```python
from build123d import *

# Parameters (mm, degrees)
SKETCH133_W     = 50
SKETCH133_H     = 100
SKETCH133_R     = 1.9
SKETCH133_R_2   = 1.75
PAD079_DEPTH    = 10
SKETCH143_R     = 2.5
POCKET049_DEPTH = 2
SKETCH149_R     = 1.73
POCKET051_DEPTH = 10


with BuildPart() as part:
    # Sketch133 → Pad079 (new body)
    with BuildSketch(Plane.XY):
        Rectangle(SKETCH133_W, SKETCH133_H)
        with Locations((-10, 40)):
            Circle(SKETCH133_R, mode=Mode.SUBTRACT)
        with Locations((10, 40)):
            Circle(SKETCH133_R, mode=Mode.SUBTRACT)
        with Locations((10, 20)):
            Circle(SKETCH133_R, mode=Mode.SUBTRACT)
        with Locations((-10, 20)):
            Circle(SKETCH133_R, mode=Mode.SUBTRACT)
        with Locations((-10, -20)):
            Circle(SKETCH133_R, mode=Mode.SUBTRACT)
        with Locations((10, -20)):
            Circle(SKETCH133_R, mode=Mode.SUBTRACT)
        with Locations((10, -40)):
            Circle(SKETCH133_R, mode=Mode.SUBTRACT)
        with Locations((-10, -40)):
            Circle(SKETCH133_R, mode=Mode.SUBTRACT)
        with Locations((12.5, 0)):
            Circle(SKETCH133_R_2, mode=Mode.SUBTRACT)
        with Locations((-12.5, 0)):
            Circle(SKETCH133_R_2, mode=Mode.SUBTRACT)
        with Locations((20, 40)):
            Circle(SKETCH133_R_2, mode=Mode.SUBTRACT)
        with Locations((20, 20)):
            Circle(SKETCH133_R_2, mode=Mode.SUBTRACT)
        with Locations((-20, 40)):
            Circle(SKETCH133_R_2, mode=Mode.SUBTRACT)
        with Locations((-20, 20)):
            Circle(SKETCH133_R_2, mode=Mode.SUBTRACT)
        with Locations((-20, -20)):
            Circle(SKETCH133_R_2, mode=Mode.SUBTRACT)
        with Locations((-20, -40)):
            Circle(SKETCH133_R_2, mode=Mode.SUBTRACT)
        with Locations((20, -20)):
            Circle(SKETCH133_R_2, mode=Mode.SUBTRACT)
        with Locations((20, -40)):
            Circle(SKETCH133_R_2, mode=Mode.SUBTRACT)
    extrude(amount=PAD079_DEPTH)

    # Sketch143 → Pocket049 (cut)
    with BuildSketch(Plane.YZ.offset(25)):
        with Locations((-45, 5)):
            Circle(SKETCH143_R)
        with Locations((45, 5)):
            Circle(SKETCH143_R)
    extrude(amount=-POCKET049_DEPTH, mode=Mode.SUBTRACT)

    # Sketch149 → Pocket051 (cut)
    with BuildSketch(Plane.YZ.offset(-25)):
        with Locations((-10, 5)):
            Circle(SKETCH149_R)
        with Locations((10, 5)):
            Circle(SKETCH149_R)
    extrude(amount=POCKET051_DEPTH, mode=Mode.SUBTRACT)


solid = part.part
```
The model under review builds one solid part; all positions refer to its coordinate system, in mm. A direction names the side the tool comes from. Coordinates: 2 decimals unless noted, no trailing zeros. Write each loop counter-clockwise with the first axis right and the second up, starting at its lowest first coordinate (ties: lowest second). Pieces come first, ordered by that corner, then holes. Notation, with made-up numbers: (57.25, 37.5) -> (73.25, 37.5) arc R24 cw to (73.25, 47.5) -> close; hole circle Ø9 at (-7, 10.5). An arc over 180 degrees is marked (long way). One line per item, written item: value. Start each with the question number.
Q1. Add section C-C, the plane x = 20. Give the boundary of the cut face in (y, z).
Q2. Add section B-B, the plane y = 20. Give the boundary of the cut face in (x, z), then the cut area to 3 significant figures.
Q3. Add section A-A, the plane x = -20. Give the boundary of the cut face in (y, z), then the cut area to 3 significant figures.
Q4. For faces 1 (the face through (23, 45, 5)), 2 (the face through (-15, -10, 5)), 3 (the face through (0, 50, 5)), list the 3-axis set-ups (+Z, -Z, +X, -X, +Y, -Y) from which the entire face can be reached by the end or side of a thin tool; tool diameter is ignored.
Q5. To check wall thickness, follow probe 1 along Y at (x, z) = (10, 6); probe 2 along Y at (x, z) = (20, 3.25); probe 3 along Y at (x, z) = (12.5, 5.25). State the ranges of each line that lie inside material, in increasing order.
Q6. Add section D-D, the plane y = 10. Give the boundary of the cut face in (x, z), then the cut area to 3 significant figures.
Q7. Clearance check with flat-ended pins moving along their axes: P1, Ø3, axis at y = -10, z = 5, coming from the -X side; P2, Ø1.5, axis at y = -44.5, z = 4, coming from the +X side. State where each tip first meets the part, or that it passes through.
Q8. The part is to be moulded in two halves that separate along Z. For faces 4 (the face through (24.01, 47.31, 4.04)), 5 (the face through (0, 1, 10)), 6 (the face through (18.61, 38.94, 4.93)), 7 (the face through (0, 1, 0)), say which applies: +Z half, -Z half, draft (parallel to the pull), parting line (faces both ways), or undercut.
Response:
1. outline: (-50, 0) -> (-41.75, 0) -> (-41.75, 10) -> (-50, 10) -> close; (-38.25, 0) -> (-21.75, 0) -> (-21.75, 10) -> (-38.25, 10) -> close; (-18.25, 0) -> (18.25, 0) -> (18.25, 10) -> (-18.25, 10) -> close; (21.75, 0) -> (38.25, 0) -> (38.25, 10) -> (21.75, 10) -> close; (41.75, 0) -> (50, 0) -> (50, 10) -> (41.75, 10) -> close
2. outline: (-25, 0) -> (-21.75, 0) -> (-21.75, 10) -> (-25, 10) -> close; (-18.25, 0) -> (-11.9, 0) -> (-11.9, 10) -> (-18.25, 10) -> close; (-8.1, 0) -> (8.1, 0) -> (8.1, 10) -> (-8.1, 10) -> close; (11.9, 0) -> (18.25, 0) -> (18.25, 10) -> (11.9, 10) -> close; (21.75, 0) -> (25, 0) -> (25, 10) -> (21.75, 10) -> close
2. area: 354 mm²
3. outline: (-50, 0) -> (-41.75, 0) -> (-41.75, 10) -> (-50, 10) -> close; (-38.25, 0) -> (-21.75, 0) -> (-21.75, 10) -> (-38.25, 10) -> close; (-18.25, 0) -> (18.25, 0) -> (18.25, 10) -> (-18.25, 10) -> close; (21.75, 0) -> (38.25, 0) -> (38.25, 10) -> (21.75, 10) -> close; (41.75, 0) -> (50, 0) -> (50, 10) -> (41.75, 10) -> close; hole circle Ø3.46 at (-10, 5); hole circle Ø3.46 at (10, 5)
3. area: 841 mm²
4. face 1: +X
4. face 2: -X
4. face 3: +Z, -Z, +X, -X, +Y
5. probe 1: -50 to -41.9, -38.1 to -21.9, -18.1 to 18.1, 21.9 to 38.1, 41.9 to 50
5. probe 2: -50 to -41.75, -38.25 to -21.75, -18.25 to 18.25, 21.75 to 38.25, 41.75 to 50
5. probe 3: -50 to -1.75, 1.75 to 50
6. outline: (-25, 0) -> (25, 0) -> (25, 10) -> (-25, 10) -> (-25, 6.73) -> (-15, 6.73) -> (-15, 3.27) -> (-25, 3.27) -> close
6. area: 465 mm²
7. P1: x = -15
7. P2: x = 23
8. face 4: undercut
8. face 5: +Z half
8. face 6: draft
8. face 7: -Z half
